CAD build for the part. Positions are in the model's coordinates, mm. A direction names the side the tool comes from. Give positions to 0.01 mm unless a question says otherwise; leave off trailing zeros. Write each loop counter-clockwise with the first axis right and the second up, starting at its lowest first coordinate (ties: lowest second). Pieces come first, ordered by that corner, then holes. Notation, with made-up numbers: (37, 19) - (90, 19) arc R23 cw to (90, 37) - close; hole circle Ø8 at (48, -3.5). An arc over 180 degrees is marked (long way). Answer as a JSON object with one key per item and string values.
from build123d import *

# Parameters (mm, degrees)
SKETCH1_W             = 12.75
SKETCH1_H             = 12.75
BOSS_EXTRUDE1_DEPTH   = 2
SKETCH2_W             = 12.75
SKETCH2_H             = 12.75
BOSS_EXTRUDE2_DEPTH   = 2
SKETCH3_W             = 12.75
SKETCH3_H             = 10
BOSS_EXTRUDE3_DEPTH   = 2
F_1_0MM_DOWEL_HOLE1_D = 1.75
F_1_0MM_DOWEL_HOLE2_D = 1.5


with BuildPart() as part:
    # Sketch1 → Boss-Extrude1 (new body)
    with BuildSketch(Plane.XY):
        with Locations((-6.375, 6.375)):
            Rectangle(SKETCH1_W, SKETCH1_H)
    extrude(amount=BOSS_EXTRUDE1_DEPTH)



with BuildPart() as body_2:
    # Sketch2 → Boss-Extrude2 (new body)
    with BuildSketch(Plane(origin=(0, 0, -6), x_dir=(-1, 0, 0), z_dir=(0, 0, -1))):
        with Locations((6.375, 6.375)):
            Rectangle(SKETCH2_W, SKETCH2_H)
    extrude(amount=BOSS_EXTRUDE2_DEPTH)


with BuildPart() as part_1:
    add(part.part)

    add(body_2.part)  # Boss-Extrude3 merges body 2
    # Sketch3 → Boss-Extrude3 (add)
    with BuildSketch(Plane(origin=(0, 12.75, 0), x_dir=(1, 0, 0), z_dir=(0, 1, 0))):
        with Locations((-6.375, 3)):
            Rectangle(SKETCH3_W, SKETCH3_H)
    extrude(amount=BOSS_EXTRUDE3_DEPTH)

    # Ø1.0mm Dowel Hole1 (through all)
    with Locations(Plane.XY.offset(2)):
        with Locations((-9.375, 4), (-3.375, 4)):
            Hole(F_1_0MM_DOWEL_HOLE1_D / 2)

    # Ø1.0mm Dowel Hole2 (through all)
    with Locations(Plane(origin=(0, 14.75, 0), x_dir=(1, 0, 0), z_dir=(0, 1, 0))):
        with Locations((-8.75, 3)):
            Hole(F_1_0MM_DOWEL_HOLE2_D / 2)


solid = part_1.part
Item 1: Cut at A-A (y = 4). Give the cut face in (x, z), and give its area (3 significant figures).
Entries:
{"outline": "(-12.75, -8) - (-10.25, -8) - (-10.25, -6) - (-12.75, -6) - close; (-12.75, 0) - (-10.25, 0) - (-10.25, 2) - (-12.75, 2) - close; (-8.5, -8) - (-4.25, -8) - (-4.25, -6) - (-8.5, -6) - close; (-8.5, 0) - (-4.25, 0) - (-4.25, 2) - (-8.5, 2) - close; (-2.5, -8) - (0, -8) - (0, -6) - (-2.5, -6) - close; (-2.5, 0) - (0, 0) - (0, 2) - (-2.5, 2) - close", "area": "37.0 mm2"}
Item 2: Mould opens along X. For faces 1 (the flat face through (-12.75, 7.3, -6.3)), 2 (the flat face through (-6, 6, 0)), 3 (the cylindrical face through (-8, 14, -3)) say: +X half, -X half, draft (parallel to the pull), parting line (faces both ways), or undercut.
Entries:
{"face 1": "-X half", "face 2": "draft", "face 3": "undercut"}
Item 3: Probe line 1 (Z direction, x = -5.5, y = 9.25); line 2 (Z direction, x = -8.75, y = 13.6); line 3 (Y direction, x = -5.25, z = -5.75). List the from-to ranges inside material, lowest first. Write a range as from..to.
Entries:
{"line 1": "-8..-6, 0..2", "line 2": "-8..-3.75, -2.25..2", "line 3": "12.75..14.75"}
Item 4: Flat gauge pin, fed straight in: P1, Ø1.4, axis at x = -8.75, z = -3, coming from the -Y side. Where does the tip first touch, or does it go through?
Entries:
{"P1": "through"}
Item 5: Which spindle directions (+Z, -Z, +X, -X, +Y, -Y) get a long thin tool onto all of the face, cutting with end or side? Do faces 4 (the flat face through (-6, 12.75, -3)), 5 (the cylindrical face through (-3.261, 4.868, -7.014)). Say none if no direction does.
Entries:
{"face 4": "+X, -X, -Y", "face 5": "+Z, -Z"}
Item 6: Cut at D-D (y = 6.5). Give the cut face in (x, z).
Entries:
{"outline": "(-12.75, -8) - (0, -8) - (0, -6) - (-12.75, -6) - close; (-12.75, 0) - (0, 0) - (0, 2) - (-12.75, 2) - close"}
Item 7: Cut at C-C (x = -8.75). Give the cut face in (y, z).
Entries:
{"outline": "(0, -8) - (3.39, -8) - (3.39, -6) - (0, -6) - close; (0, 0) - (3.39, 0) - (3.39, 2) - (0, 2) - close; (4.61, -8) - (14.75, -8) - (14.75, -3.75) - (12.75, -3.75) - (12.75, -6) - (4.61, -6) - close; (4.61, 0) - (12.75, 0) - (12.75, -2.25) - (14.75, -2.25) - (14.75, 2) - (4.61, 2) - close"}
Item 8: Cut at B-B (z = -3). Give the cut face in (x, y), and give its area (3 significant figures).
Entries:
{"outline": "(-12.75, 12.75) - (-9.5, 12.75) - (-9.5, 14.75) - (-12.75, 14.75) - close; (-8, 12.75) - (0, 12.75) - (0, 14.75) - (-8, 14.75) - close", "area": "22.5 mm2"}
